from build123d import *
from OCP.BRepFilletAPI import BRepFilletAPI_MakeChamfer

# Parameters (mm, degrees)
CHAMFER_1_SIZE      = 0.2
CHAMFER_1_SIZE2     = 0.6
CUT_EXTRUDE_1_DEPTH = 6.622206177
SKETCH_3_R          = 13
CUT_EXTRUDE_3_DEPTH = 23.650187091


with BuildPart() as part:
    # 草图1 → 旋转1 (revolve)
    with BuildSketch(Plane.XY, mode=Mode.PRIVATE) as revolve_1_sk:
        with BuildLine():
            Line((6, 19.622206177), (3, 19.622206177))
            Line((3, 19.622206177), (3, 6.622206177))
            Line((3, 6.622206177), (0, 6.622206177))
            Line((0, 6.622206177), (0, 3))
            Line((0, 3), (5.45, 3))
            Line((5.45, 3), (5.45, 0))
            Line((5.45, 0), (6.45, 0))
            Line((6.45, 0), (6.45, 8))
            Line((6.45, 8), (8, 8))
            Line((8, 8), (8, 13.122206177))
            Line((8, 13.122206177), (6, 13.122206177))
            Line((6, 13.122206177), (6, 13.622206177))
            ThreePointArc((6, 13.622206177), (5.596229956, 15.079944151), (4.5, 16.122206177))
            Line((4.5, 16.122206177), (4, 16.122206177))
            Line((4, 16.122206177), (4, 16.622206177))
            Line((4, 16.622206177), (3.5, 16.622206177))
            Line((3.5, 16.622206177), (3.5, 17.622206177))
            Line((3.5, 17.622206177), (6, 17.622206177))
            Line((6, 17.622206177), (6, 19.622206177))
        make_face()
    revolve(revolve_1_sk.sketch.rotate(Axis((0, 26.759420291, 0), (0, -1, 0)), 90), axis=Axis((0, 26.759420291, 0), (0, -1, 0)))

    # 倒角1: one chamfer whose edges measure the first distance from different faces: ONE call of the kernel's chamfer builder (chamfer() names one face for all edges)
    chamfer_1_edges_1 = [part.edges().sort_by_distance(p)[0] for p in [
        (0, 13.122206177, -8),
    ]]
    chamfer_1_side_1 = [part.faces().sort_by_distance(p)[0] for p in [
        (0, 10.561103089, -8),
    ]]
    chamfer_1_edges_2 = [part.edges().sort_by_distance(p)[0] for p in [
        (0, 8, -8),
    ]]
    chamfer_1_side_2 = [part.faces().sort_by_distance(p)[0] for p in [
        (0, 8, -6.67627417),
    ]]
    chamfer_1 = BRepFilletAPI_MakeChamfer(part.part.solid().wrapped)
    for e in chamfer_1_edges_1:
        chamfer_1.Add(CHAMFER_1_SIZE, CHAMFER_1_SIZE2, e.wrapped, chamfer_1_side_1[0].wrapped)  # the first distance lies on this face
    for e in chamfer_1_edges_2:
        chamfer_1.Add(CHAMFER_1_SIZE, CHAMFER_1_SIZE2, e.wrapped, chamfer_1_side_2[0].wrapped)  # the first distance lies on this face
    add(Compound.cast(chamfer_1.Shape()), mode=Mode.REPLACE)

    # 草图2 → 切除-拉伸1 (cut)
    with BuildSketch(Plane(origin=(0, 0, 0), x_dir=(1, 0, 0), z_dir=(0, 1, 0))):
        Polygon((2, 1.154700538), (0, 2.309401077), (-2, 1.154700538), (-2, -1.154700538), (0, -2.309401077), (2, -1.154700538), align=None)
    extrude(amount=CUT_EXTRUDE_1_DEPTH, mode=Mode.SUBTRACT)

    # 草图3 → 切除-拉伸3 (cut, through all)
    with BuildSketch(Plane(origin=(0, 0, 0), x_dir=(1, 0, 0), z_dir=(0, 1, 0))):
        Circle(SKETCH_3_R)
        Polygon((8, 0), (4, 6.92820323), (-4, 6.92820323), (-8, 0), (-4, -6.92820323), (4, -6.92820323), align=None, mode=Mode.SUBTRACT)
    extrude(amount=CUT_EXTRUDE_3_DEPTH, mode=Mode.SUBTRACT)


solid = part.part
Geometry: final body of the model. Coordinates: model frame, mm. A direction names the side the tool comes from. Round coordinates to 2 decimals unless told otherwise and drop trailing zeros. Loops run counter-clockwise (first coordinate to the right, second up) from the corner with the lowest first, then second, coordinate; pieces in that order, holes last. Notation, with made-up numbers: M -27.75,-21.75 L 17.25,-21.75 A25 cw 17.25,2.25 Z; hole C 33,32 d2. An arc over 180 degrees is marked long. Put each result on its own line as item: value. Start each with the question number.
(1) Section query A-A (y = 9). Return loops of the section in (x, z).
(2) Set-up query: faces 1 (the face through (5.72, 4.06, 2.98)), 2 (the face through (2, 5, 0)), 3 (the face through (-1.802, 18.636, 5.723)), 4 (the face through (1, 19.622, -3)), 5 (the face through (3.105, 17.129, 1.615)). Return all of +Z, -Z, +X, -X, +Y, -Y with unobstructed straight access to the full face (end or side cutting, diameter ignored); none if empty.
(3) Section query C-C (y = 18). Return loops of the section in (x, z).
(4) Draft query along X for faces 6 (the face through (-2, 5, 0)), 7 (the face through (3.905, 16.376, -0.867)), 8 (the face through (3.796, 13.068, 6.541)). Return one class per face: +X half, -X half, draft (parallel to the pull), parting line (faces both ways), or undercut.
(5) Material intervals for line 1 along Y through (x, z) = (1.5, 4); line 2 along X through (y, z) = (4.25, 0); line 3 along X through (y, z) = (1.7, 0), sorted ascending. Write a range as [from, to].
(6) Section query B-B (y = 4). Return loops of the section in (x, z), then the cut area to 3 significant figures.
(7) Contact query for flat-ended pins moving along their axis: pin 1 Ø2 at (x, z) = (-2.5, 2) entering from -Y; pin 2 Ø1.2 at (y, z) = (5, 0.5) entering from -X; pin 3 Ø2 at (x, y) = (6, 5) entering from -Z. Output: stop coordinate, or through.
Findings below:
1. outline: M -8,0 L -4,-6.93 L 4,-6.93 L 8,0 L 4,6.93 L -4,6.93 Z; hole C 0,0 d6
2. face 1: -Y
2. face 2: +Y, -Y
2. face 3: +Y
2. face 4: +Z, -Z, +X, -X, +Y
2. face 5: none
3. outline: C 0,0 d12; hole C 0,0 d6
4. face 6: undercut
4. face 7: parting line
4. face 8: +X half
5. line 1: y = [3, 16.12], [17.62, 19.62]
5. line 2: x = [-6.45, -2], [2, 6.45]
5. line 3: x = [-6.45, -5.45], [5.45, 6.45]
6. outline: C 0,0 d12.9; hole M -2,-1.15 L 0,-2.31 L 2,-1.15 L 2,1.15 L 0,2.31 L -2,1.15 Z
6. area: 117 mm2
7. pin 1: stops at y = 3
7. pin 2: stops at x = -6.45
7. pin 3: stops at z = -4.07
